Input: dimensioned drawing with shaded views. Units: mm. Origin: part minimum x, y, z. A direction names the side the tool comes from. Round coordinates to 2 decimals unless told otherwise and drop trailing zeros. Order: outer loops, then holes, each group sorted by start corner. A loop starts at its lowest first (then second) coordinate and runs counter-clockwise, first axis right, second up.
Item 1: Reachability of the marked faces 1 and 2 from +Z, -Z, +X, -X, +Y, -Y: full face, straight path, thin tool, end or side. Return the list, or none.
Item 2: First-contact query: pin 1 (10 mm diameter, centred on x = 12.7, y = 9.525, fed in from +Z); pin 2 (3 mm diameter, centred on x = 7.5, y = 10, fed in from +Z); pin 3 (6 mm diameter, centred on x = 12.7, z = 15.875, fed in from -Y); pin 4 (14 mm diameter, centred on x = 15.5, z = 14, fed in from -Y). Flat tips, straight axial feed; report the tip coordinate or a pass-through.
Item 3: Line query: L1, parallel to Z at x = 12.7, y = 23.5 (3 decimals); L2, parallel to Y at x = 18.75, z = 19.5; L3, parallel to Z at x = 2.5, y = 13.25. Output: solid intervals per line, ascending.
Item 4: Cut plane B-B on y = 6.5. Output: boundary loops of the cut face in (x, z), then the cut area to 3 significant figures.
Item 5: Cut plane D-D on x = 2.75. Output: boundary loops of the cut face in (y, z) (3 decimals), then the cut area to 3 significant figures.
Item 6: Cut plane C-C on z = 14. Output: boundary loops of the cut face in (x, y).
Item 7: Cut plane A-A on x = 12.7. Output: boundary loops of the cut face in (y, z) (3 decimals), then the cut area to 3 significant figures.
Item 8: Mould query, pull axis X, two halves, no side actions, for the marked faces 3, 4, 5 and 6. Classes: released by +X, released by -X, zero draft, split by the parting line, or undercut.
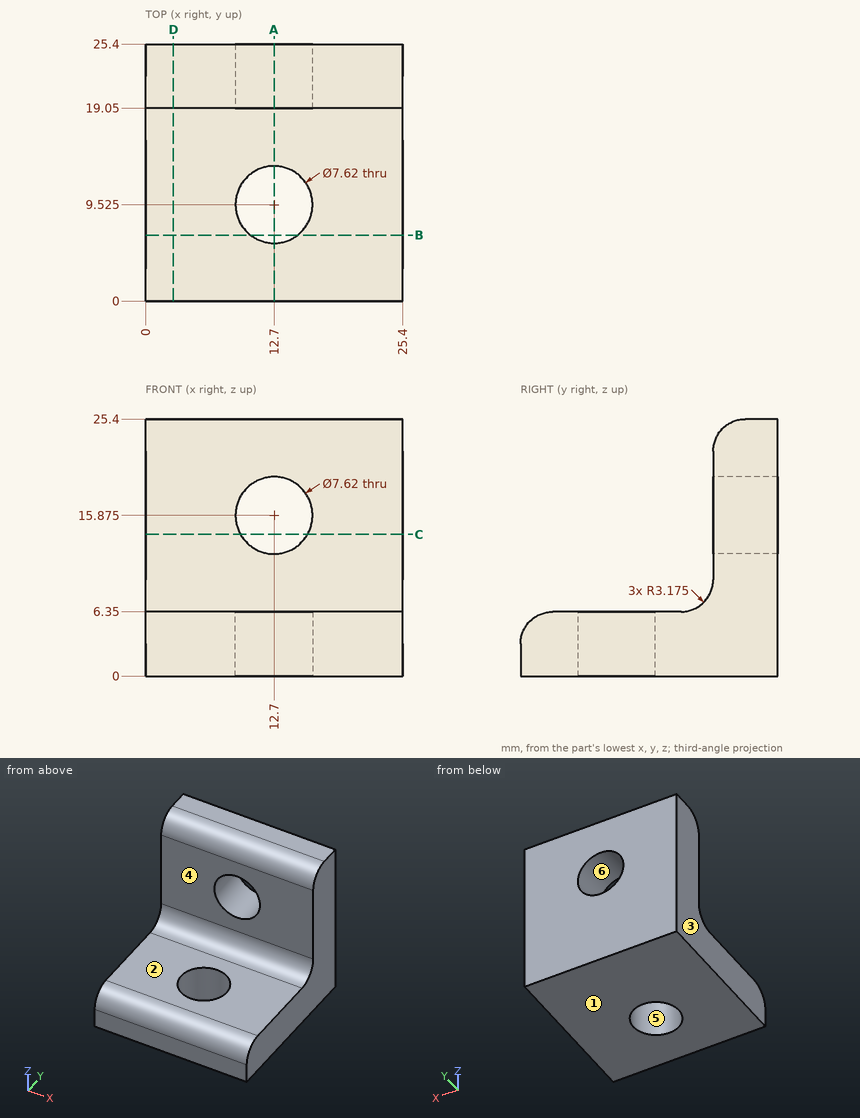
From the geometry:
1. face 1: -Z, +X, -X, +Y, -Y
1. face 2: +Z, +X, -X, -Y
2. pin 1: stops at z = 6.35
2. pin 2: stops at z = 6.35
2. pin 3: passes through
2. pin 4: stops at y = 17.8
3. L1: z = 0 to 12.065, 19.685 to 25.4
3. L2: y = 19.05 to 25.4
3. L3: z = 0 to 6.35
4. outline: (0, 0) - (10.38, 0) - (10.38, 6.35) - (0, 6.35) - close; (15.02, 0) - (25.4, 0) - (25.4, 6.35) - (15.02, 6.35) - close
4. area: 132 mm2
5. outline: (0, 0) - (25.4, 0) - (25.4, 25.4) - (22.225, 25.4) arc R3.175 ccw to (19.05, 22.225) - (19.05, 9.525) arc R3.175 cw to (15.875, 6.35) - (3.175, 6.35) arc R3.175 ccw to (0, 3.175) - close
5. area: 280 mm2
6. outline: (0, 19.05) - (9.38, 19.05) - (9.38, 25.4) - (0, 25.4) - close; (16.02, 19.05) - (25.4, 19.05) - (25.4, 25.4) - (16.02, 25.4) - close
7. outline: (0, 0) - (5.715, 0) - (5.715, 6.35) - (3.175, 6.35) arc R3.175 ccw to (0, 3.175) - close; (13.335, 0) - (25.4, 0) - (25.4, 12.065) - (19.05, 12.065) - (19.05, 9.525) arc R3.175 cw to (15.875, 6.35) - (13.335, 6.35) - close; (19.05, 19.685) - (25.4, 19.685) - (25.4, 25.4) - (22.225, 25.4) arc R3.175 ccw to (19.05, 22.225) - close
7. area: 183 mm2
8. face 3: released by -X
8. face 4: zero draft
8. face 5: undercut
8. face 6: undercut
